```python
from build123d import *

# Parameters (mm, degrees)
F0_W        = 100
F0_H        = 100
F0_W_2      = 190
F0_H_2      = 550
F1_DEPTH    = 550
F3_DEPTH    = 190
F4_T        = 2.5
F4_T3_DEPTH = 105
F4_T5_DEPTH = 105
F6_DEPTH    = 98.5
F7_W        = 185
F7_H        = 5
F8_DEPTH    = 2.5
F9_DEPTH    = 1099


# Not quite as in the source:
# - a shell that OpenCascade refuses in one call is made with other operations: the cavity is built on its own and cut out


with BuildPart() as f1:
    # F0 (on Front) → F1 (new body, symmetric)
    with BuildSketch(Plane.XZ):
        with Locations((0, -450)):
            Rectangle(F0_W, F0_H)
        with Locations((0, 275)):
            Rectangle(F0_W_2, F0_H_2)
        Polygon((50, -400), (95, 0), (-95, 0), (-50, -400), align=None)
    extrude(amount=F1_DEPTH, both=True)

    # F2 (on face) → F3 (cut)
    with BuildSketch(Plane.YZ.offset(95)):
        Polygon((550, -500), (550, 0), (-450, -400), (-450, -500), align=None)
    extrude(amount=-F3_DEPTH, mode=Mode.SUBTRACT)

    # F4: shell of thickness 2.5, made by hand


with BuildPart() as f4_core1:
    # F4_t2: copy of F1
    add(f1.part)

    # the walls: a layer under each face that stays
    f4_faces = [f4_core1.faces().sort_by_distance(p)[0] for p in [
        (50, -500, -450),
        (0, -550, 25),
        (72.5, 0, -200),
        (0, -450, -450),
        (-50, -500, -450),
        (95, 0, 275),
        (-95, 0, 275),
        (-72.5, 0, -200),
        (0, 50, -200),
        (0, 550, 275),
    ]]
    thicken(f4_faces, amount=-F4_T, mode=Mode.SUBTRACT)

    # F4_s4 → F4_t3 (cut)
    with BuildSketch(Plane.XZ.offset(447.5)):
        Polygon((50.0498432829, -400.0027948693), (47.5, -400), (47.5, -399.8598171527), (47.5156717096, -399.7205130673), align=None)
        Polygon((-50.0498432829, -400.0027948693), (-47.5, -400), (-47.5, -399.8598171527), (-47.5156717096, -399.7205130673), align=None)
    extrude(amount=F4_T3_DEPTH, mode=Mode.SUBTRACT)

    # F4_s6 → F4_t5 (cut)
    with BuildSketch(Plane.YZ.offset(-52.5)):
        Polygon((-449.9657152331, -400.0232119173), (-452.5, -400), (-452.5, -398.3074175964), (-450.9284766909, -397.6788082728), align=None)
    extrude(amount=F4_T5_DEPTH, mode=Mode.SUBTRACT)


with BuildPart() as f1_1:
    add(f1.part)

    # what is left inside the walls is the cavity
    f4_cavity = [f4_core1.part.solids().sort_by_distance(p)[0] for p in [
        (-92.475, 182.5, 275.070091),
    ]]
    add(f4_cavity, mode=Mode.SUBTRACT)

    # F5 (on face) → F6 (cut)
    with BuildSketch(Plane.XZ.offset(550)):
        Polygon((-48.5, -495), (-48.5, -500), (48.5, -500), (48.5, -495), (49.5, -495), (49.5, -490), (-49.5, -490), (-49.5, -495), align=None)
    extrude(amount=-F6_DEPTH, mode=Mode.SUBTRACT)

    # F7 (on face) → F8 (cut)
    with BuildSketch(Plane(origin=(0, 550, 0), x_dir=(-1, 0, 0), z_dir=(0, 1, 0))):
        with Locations((0, 547.5)):
            Rectangle(F7_W, F7_H)
    extrude(amount=-F8_DEPTH, mode=Mode.SUBTRACT)

    # F7 (on face) → F9 (cut)
    with BuildSketch(Plane(origin=(0, 550, 0), x_dir=(-1, 0, 0), z_dir=(0, 1, 0))):
        Polygon((92.5, 545), (-92.5, 545), (-94, 545), (-94, 540), (94, 540), (94, 545), align=None)
    extrude(amount=-F9_DEPTH, mode=Mode.SUBTRACT)


solid = f1_1.part
```
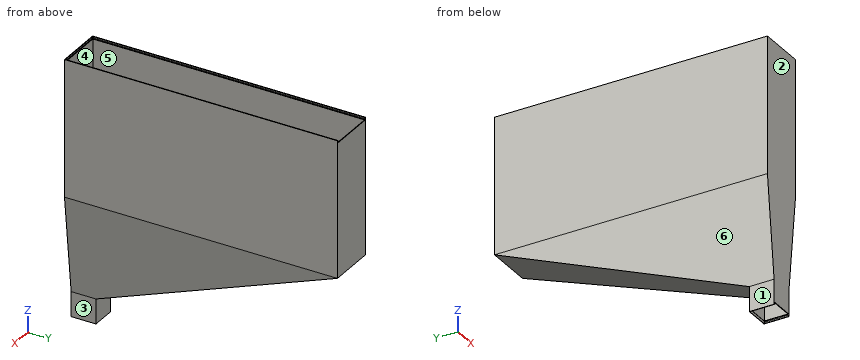
CAD build for the part. Positions are in the model's coordinates, mm. Face numbers are marked on the shaded views. A direction names the side the tool comes from. Coordinates: 2 decimals unless noted, no trailing zeros. Order: outer loops, then holes, each group sorted by start corner. A loop starts at its lowest first (then second) coordinate and runs counter-clockwise, first axis right, second up. Notation, with made-up numbers: (62.5, 9.25) - (111.5, 9.25) arc R20 ccw to (111.5, 42.25) - close; hole circle Ø5 at (10.5, 50.5). An arc over 180 degrees is marked (long way). Answer in a Markdown table with one row per item.
1. 3-axis set-ups, long thin cutter, end or side, ignore diameter. For the marked faces 1 and 2: which of +Z, -Z, +X, -X, +Y, -Y reach the whole face in a straight line?
Answer:
| item | result |
|---|---|
| face 1 | -Z, -X, +Y, -Y |
| face 2 | +Z, -Z, +X, -X, -Y |
2. Drill centre lines: L1, parallel to Y at x = -29, z = 321.5; L2, parallel to X at y = 231, z = 383; L3, parallel to X at y = -66.5, z = -63. Where is each one in solid material? Low to high. Write a range as from..to.
Answer:
| item | result |
|---|---|
| L1 | -550..-547.5, 547.5..550 |
| L2 | -95..-92.5, 92.5..95 |
| L3 | -87.91..-85.4, 85.4..87.91 |
3. Flat gauge pins, fed straight in: P1, Ø4, axis at x = -26, z = 547, coming from the +Y side; P2, Ø8, axis at y = -224.5, z = -247, coming from the +X side; P3, Ø5, axis at x = -36.5, y = 166, coming from the +Z side. Where does each tip first touch, or does it go through?
Answer:
| item | result |
|---|---|
| P1 | y = -547.5 |
| P2 | x = 67.66 |
| P3 | z = -149.91 |
4. Slice it at B-B, the plane z = 122. List the corners of the cut face in (x, y), then the cut area to 4 significant figures.
Answer:
| item | result |
|---|---|
| outline | (-95, -550) - (95, -550) - (95, 550) - (-95, 550) - close; hole (-92.5, -547.5) - (92.5, -547.5) - (92.5, 547.5) - (-92.5, 547.5) - close |
| area | 6,425 mm² |
5. Pull direction X, two halves, no side cores. Call the marked faces 3, 4, 5 and 6: +X half, -X half, draft (parallel to the pull), parting line (faces both ways), or undercut.
Answer:
| item | result |
|---|---|
| face 3 | +X half |
| face 4 | undercut |
| face 5 | undercut |
| face 6 | -X half |
6. Slice it at A-A, the plane x = -28.5. List the corners of the cut face in (y, z), then the cut area to 3 significant figures.
Answer:
| item | result |
|---|---|
| outline | (-550, -490) - (-547.5, -490) - (-547.5, 540) - (-549, 540) - (-549, 545) - (-547.5, 545) - (-547.5, 550) - (-550, 550) - close; (-452.5, -490) - (-451.5, -490) - (-451.5, -500) - (-450, -500) - (-450, -400) - (550, 0) - (550, 540) - (547.5, 540) - (547.5, 1.69) - (-452.5, -398.31) - close |
| area | 6,880 mm² |
7. Slice it at C-C, the plane y = 389.5. List the corners of the cut face in (x, z).
Answer:
| item | result |
|---|---|
| outline | (-95, 0) - (-87.78, -64.2) - (87.78, -64.2) - (95, 0) - (95, 550) - (92.5, 550) - (92.5, 545) - (94, 545) - (94, 540) - (92.5, 540) - (92.5, 0.14) - (85.56, -61.51) - (-85.56, -61.51) - (-92.5, 0.14) - (-92.5, 540) - (-94, 540) - (-94, 545) - (-92.5, 545) - (-92.5, 550) - (-95, 550) - close |
8. Slice it at D-D, the plane z = -251.5. List the corners of the cut face in (x, y), then the cut area to 3 significant figures.
Answer:
| item | result |
|---|---|
| outline | (-66.71, -550) - (66.71, -550) - (66.71, -78.75) - (-66.71, -78.75) - close; hole (-64.19, -547.5) - (64.19, -547.5) - (64.19, -85.48) - (-64.19, -85.48) - close |
| area | 3,560 mm² |
